from build123d import *

# Parameters (mm, degrees)
F1_DEPTH = 2
F2_DEPTH = 57
F3_DEPTH = 127


with BuildPart() as f1:
    # F0 (on Front) → F1 (new body)
    with BuildSketch(Plane.XZ):
        with BuildLine():
            ThreePointArc((14.3614066163, -2), (-14.5, 0), (14.3614066163, 2))
            Line((14.3614066163, 2), (16.3783393542, 2))
            ThreePointArc((16.3783393542, 2), (-16.5, 0), (16.3783393542, -2))
            Line((16.3783393542, -2), (14.3614066163, -2))
        make_face()
        with BuildLine():
            Line((16.3783393542, 2), (14.3614066163, 2))
            ThreePointArc((14.3614066163, 2), (14.465310158, 1.0023981402), (14.5, 0))
            ThreePointArc((14.5, 0), (14.465310158, -1.0023981402), (14.3614066163, -2))
            Line((14.3614066163, -2), (16.3783393542, -2))
            ThreePointArc((16.3783393542, -2), (16.469556754, -1.0018484557), (16.5, 0))
            ThreePointArc((16.5, 0), (16.469556754, 1.0018484557), (16.3783393542, 2))
        make_face()
    extrude(amount=F1_DEPTH)

    # F0 (on Front) → F2 (join)
    with BuildSketch(Plane.XZ):
        with BuildLine():
            ThreePointArc((13.4521373766, -2), (-13.6, 0), (13.4521373766, 2))
            Line((13.4521373766, 2), (14.3614066163, 2))
            ThreePointArc((14.3614066163, 2), (-14.5, 0), (14.3614066163, -2))
            Line((14.3614066163, -2), (13.4521373766, -2))
        make_face()
        with BuildLine():
            ThreePointArc((13.4521373766, 2), (13.5629839697, 1.0027291952), (13.6, 0))
            ThreePointArc((13.6, 0), (13.5629839697, -1.0027291952), (13.4521373766, -2))
            Line((13.4521373766, -2), (14.3614066163, -2))
            ThreePointArc((14.3614066163, -2), (14.465310158, -1.0023981402), (14.5, 0))
            ThreePointArc((14.5, 0), (14.465310158, 1.0023981402), (14.3614066163, 2))
            Line((14.3614066163, 2), (13.4521373766, 2))
        make_face()
    extrude(amount=F2_DEPTH)

    # F0 (on Front) → F3 (cut)
    with BuildSketch(Plane.XZ):
        with BuildLine():
            Line((19.9760421067, 2), (16.3783393542, 2))
            ThreePointArc((16.3783393542, 2), (16.469556754, 1.0018484557), (16.5, 0))
            ThreePointArc((16.5, 0), (16.469556754, -1.0018484557), (16.3783393542, -2))
            Line((16.3783393542, -2), (19.9760421067, -2))
            Line((19.9760421067, -2), (19.9760421067, 2))
        make_face()
        with BuildLine():
            Line((16.3783393542, 2), (14.3614066163, 2))
            ThreePointArc((14.3614066163, 2), (14.465310158, 1.0023981402), (14.5, 0))
            ThreePointArc((14.5, 0), (14.465310158, -1.0023981402), (14.3614066163, -2))
            Line((14.3614066163, -2), (16.3783393542, -2))
            ThreePointArc((16.3783393542, -2), (16.469556754, -1.0018484557), (16.5, 0))
            ThreePointArc((16.5, 0), (16.469556754, 1.0018484557), (16.3783393542, 2))
        make_face()
        with BuildLine():
            ThreePointArc((13.4521373766, 2), (13.5629839697, 1.0027291952), (13.6, 0))
            ThreePointArc((13.6, 0), (13.5629839697, -1.0027291952), (13.4521373766, -2))
            Line((13.4521373766, -2), (14.3614066163, -2))
            ThreePointArc((14.3614066163, -2), (14.465310158, -1.0023981402), (14.5, 0))
            ThreePointArc((14.5, 0), (14.465310158, 1.0023981402), (14.3614066163, 2))
            Line((14.3614066163, 2), (13.4521373766, 2))
        make_face()
        with BuildLine():
            ThreePointArc((13.4521373766, -2), (13.5629839697, -1.0027291952), (13.6, 0))
            ThreePointArc((13.6, 0), (13.5629839697, 1.0027291952), (13.4521373766, 2))
            Line((13.4521373766, 2), (7.9760421067, 2))
            Line((7.9760421067, 2), (7.9760421067, -2))
            Line((7.9760421067, -2), (13.4521373766, -2))
        make_face()
    extrude(amount=F3_DEPTH, mode=Mode.SUBTRACT)


solid = f1.part
The model under review builds one solid part; all positions refer to its coordinate system, in mm. A direction names the side the tool comes from. Round coordinates to 2 decimals unless told otherwise and drop trailing zeros. Order: outer loops, then holes, each group sorted by start corner. A loop starts at its lowest first (then second) coordinate and runs counter-clockwise, first axis right, second up. Notation, with made-up numbers: (-26, -3) -> (-4, -3) arc R15 ccw to (-4, 22) -> close; hole circle Ø8 at (64, 70.5). An arc over 180 degrees is marked (long way). Return JSON: item names as keys, results as strings.
1. Take a section at A-A (x = 0). Write out the cut boundary in (y, z), then the cut area to 3 significant figures.
Answer block:
{"outline": "(-57, -14.5) -> (-2, -14.5) -> (-2, -16.5) -> (0, -16.5) -> (0, -13.6) -> (-57, -13.6) -> close; (-57, 13.6) -> (0, 13.6) -> (0, 16.5) -> (-2, 16.5) -> (-2, 14.5) -> (-57, 14.5) -> close", "area": "111 mm²"}
2. Take a section at D-D (y = -15). Write out the cut boundary in (x, z).
Answer block:
{"outline": "(13.45, -2) arc R13.6 cw (long way) to (13.45, 2) -> (14.36, 2) arc R14.5 ccw (long way) to (14.36, -2) -> close"}
3. Take a section at B-B (z = -4.5). Write out the cut boundary in (x, y), then the cut area to 3 significant figures.
Answer block:
{"outline": "(-15.87, -2) -> (-13.78, -2) -> (-13.78, -57) -> (-12.83, -57) -> (-12.83, 0) -> (-15.87, 0) -> close; (12.83, -57) -> (13.78, -57) -> (13.78, -2) -> (15.87, -2) -> (15.87, 0) -> (12.83, 0) -> close", "area": "117 mm²"}
4. The part is to be moulded in two halves that separate along Z. For faces 4 (the face through (-14, 0, -2)), 5 (the face through (-16.485, -0.986, 0.697)), 6 (the face through (14, -26, 2)), say which applies: +Z half, -Z half, draft (parallel to the pull), parting line (faces both ways), or undercut.
Answer block:
{"face 4": "draft", "face 5": "parting line", "face 6": "undercut"}
5. Insertion check: P1, Ø1.5, axis at x = 8.5, y = -10, coming from the +Z side; P2, Ø6, axis at y = -10.5, z = -11, coming from the -X side; P3, Ø5, axis at x = 1, z = -11, coming from the +Y side; P4, Ø12, axis at x = -9, y = -39.5, coming from the +Z side. Each pin has a flat end and moves straight along its axis. Give the tip position at first contact, or say it passes through.
Answer block:
{"P1": "stops at z = 12.26", "P2": "stops at x = -12.09", "P3": "passes through", "P4": "stops at z = 14.19"}
6. Take a section at C-C (z = 0). Write out the cut boundary in (x, y).
Answer block:
{"outline": "(-16.5, -2) -> (-14.5, -2) -> (-14.5, -57) -> (-13.6, -57) -> (-13.6, 0) -> (-16.5, 0) -> close"}
7. For faces 1 (the face through (-10, -57, -10)), 2 (the face through (14, -26, -2)), 3 (the face through (-14.487, -29.115, 0.609)), list the 3-axis set-ups (+Z, -Z, +X, -X, +Y, -Y) from which the entire face can be reached by the end or side of a thin tool; tool diameter is ignored.
Answer block:
{"face 1": "+Z, -Z, +X, -X, -Y", "face 2": "+X, +Y, -Y", "face 3": "-Y"}
8. For L1, parallel to Z at x = 0, y = -17.5; L2, parallel to Z at x = -5.5, y = -40; L3, parallel to X at y = -42.5, z = 8, list the stretches that pass through material, from the lowest coordinate up. Write a range as [from, to].
Answer block:
{"L1": "z = [-14.5, -13.6], [13.6, 14.5]", "L2": "z = [-13.42, -12.44], [12.44, 13.42]", "L3": "x = [-12.09, -11], [11, 12.09]"}
